Study the drawing (mm; zero at the part's minimum x, y, z) and answer. A direction names the side the tool comes from. Coordinates: 2 decimals unless noted, no trailing zeros. Loops run counter-clockwise (first coordinate to the right, second up) from the corner with the lowest first, then second, coordinate; pieces in that order, holes last. Notation, with made-up numbers: (56, 87) - (107, 87) arc R9 ccw to (107, 104) - close; hole circle Ø5 at (-35, 52.25). An arc over 180 degrees is marked (long way). Use one line per item in the form item = value. Start each with the question number.
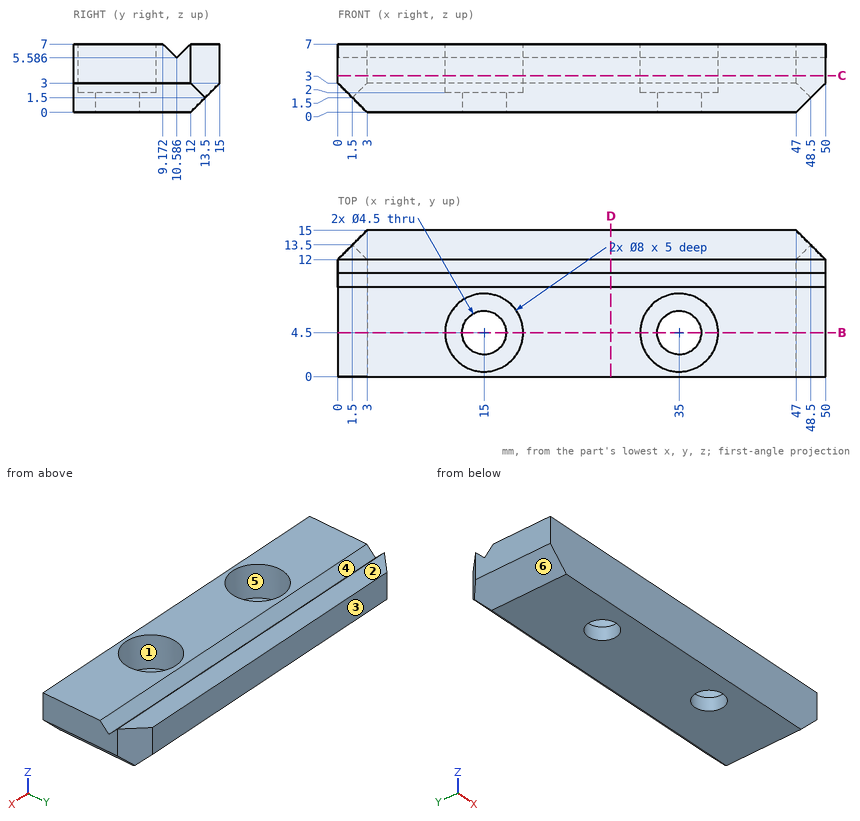
(1) Find the intervals of material crossed by probe 1 along X at (y, z) = (3, 4.75); probe 2 along X at (y, z) = (2.75, 4.75); probe 3 along Y at (x, z) = (15, 4.75), in increasing order. Write a range as from..to.
(2) For the marked faces 4, 5 and 6, determine the directions among +Z, -Z, +X, -X, +Y, -Y from which every point of the face is accessible in a straight line to the end or side of a thin tool.
(3) Determine the mould class of the marked faces 1, 2 and 3 for opening direction Y: +Y half, -Y half, draft (parallel to the pull), parting line (faces both ways), or undercut.
(4) A cutting plane is placed at C-C (z = 3.75). Determine the outline of the cut face in (x, y).
(5) Each of these flat-tipped pins is pushed along its axis until it touches: pin 1 Ø2.5 at (x, y) = (33.5, 5.5) entering from +Z; pin 2 Ø1 at (x, z) = (17.5, 2) entering from +Y. Where does it stop, or does it pass through?
(6) A cutting plane is placed at B-B (y = 4.5). Determine the outline of the cut face in (x, z).
(7) A cutting plane is placed at D-D (x = 28). Determine the outline of the cut face in (y, z) (1 decimal).
Evaluation:
q1.probe_1 = 0..11.29, 18.71..31.29, 38.71..50
q1.probe_2 = 0..11.4, 18.6..31.4, 38.6..50
q1.probe_3 = 0..0.5, 8.5..15
q2.face_4 = +Z, +X, -X
q2.face_5 = +Z
q2.face_6 = -Z, -X, +Y, -Y
q3.face_1 = undercut
q3.face_2 = draft
q3.face_3 = +Y half
q4.outline = (0, 0) - (50, 0) - (50, 12) - (47, 15) - (3, 15) - (0, 12) - close; hole circle Ø8 at (15, 4.5); hole circle Ø8 at (35, 4.5)
q5.pin_1 = 2
q5.pin_2 = 14.5
q6.outline = (0, 3) - (3, 0) - (12.75, 0) - (12.75, 2) - (11, 2) - (11, 7) - (0, 7) - close; (17.25, 0) - (32.75, 0) - (32.75, 2) - (31, 2) - (31, 7) - (19, 7) - (19, 2) - (17.25, 2) - close; (37.25, 0) - (47, 0) - (50, 3) - (50, 7) - (39, 7) - (39, 2) - (37.25, 2) - close
q7.outline = (0, 0) - (12, 0) - (15, 3) - (15, 7) - (12, 7) - (10.6, 5.6) - (9.2, 7) - (0, 7) - close
